```python
from build123d import *

# Parameters (mm, degrees)
BOSS_EXTRUDE1_DEPTH = 31.75


with BuildPart() as part:
    # Sketch1 → Boss-Extrude1 (new body)
    with BuildSketch(Plane.XY):
        Polygon((-3.579571669, 0), (-1.789785834, -3.1), (1.789785834, -3.1), (3.579571669, 0), (1.789785834, 3.1), (-1.789785834, 3.1), align=None)
    extrude(amount=BOSS_EXTRUDE1_DEPTH)

    # Sketch3 → #6-32 Tapped Hole1 (revolve, cut)
    with BuildSketch(Plane.YZ):
        Polygon((0, 0), (0, 31.75), (1.849999983, 31.75), (1.35255, 31.252550017), (1.35255, 0.497449983), (1.849999983, 0), align=None)
    revolve(axis=Axis((0, 0, -6.35), (0, 0, 1)), mode=Mode.SUBTRACT)


solid = part.part
```
Verification items for the finished model (mm, model axes). Round coordinates to 2 decimals unless told otherwise and drop trailing zeros. Order: outer loops, then holes, each group sorted by start corner. A loop starts at its lowest first (then second) coordinate and runs counter-clockwise, first axis right, second up.
1) Cross-section at A-A, the plane z = 23. Record the cut outline in (x, y).
Geometry says:
outline: (-3.58, 0) - (-1.79, -3.1) - (1.79, -3.1) - (3.58, 0) - (1.79, 3.1) - (-1.79, 3.1) - close; hole circle Ø2.71 at (0, 0)
2) Material ranges on line 1 (Y direction, x = 0, z = 27.5); line 2 (X direction, y = -0.75, z = 30.5); line 3 (X direction, y = -1, z = 9), recorded low to high.
Geometry says:
line 1: y = -3.1 to -1.35, 1.35 to 3.1
line 2: x = -3.15 to -1.13, 1.13 to 3.15
line 3: x = -3 to -0.91, 0.91 to 3
3) Cross-section at C-C, the plane x = -3. Record the cut outline in (y, z), plus the area to 3 significant figures.
Geometry says:
outline: (-1, 0) - (1, 0) - (1, 31.75) - (-1, 31.75) - close
area: 63.7 mm2
4) Draft check along Y on faces 1 (the flat face through (2, 1, 0)), 2 (the flat face through (-2.672, 1.572, 15.653)), 3 (the cylindrical face through (-0.41, 1.29, 15.66)). Enter one of: +Y half, -Y half, draft (parallel to the pull), parting line (faces both ways), or undercut.
Geometry says:
face 1: draft
face 2: +Y half
face 3: undercut
5) Cross-section at B-B, the plane x = 0. Record the cut outline in (y, z).
Geometry says:
outline: (-3.1, 0) - (-1.85, 0) - (-1.35, 0.5) - (-1.35, 31.25) - (-1.85, 31.75) - (-3.1, 31.75) - close; (1.35, 0.5) - (1.85, 0) - (3.1, 0) - (3.1, 31.75) - (1.85, 31.75) - (1.35, 31.25) - close
6) Depth check by flat-ended pin: pin 1 (1 mm diameter, centred on x = 2.5, z = 3.5, fed in from -Y). Enter the tip coordinate at first touch or a pass-through.
Geometry says:
pin 1: stops at y = -2.74
